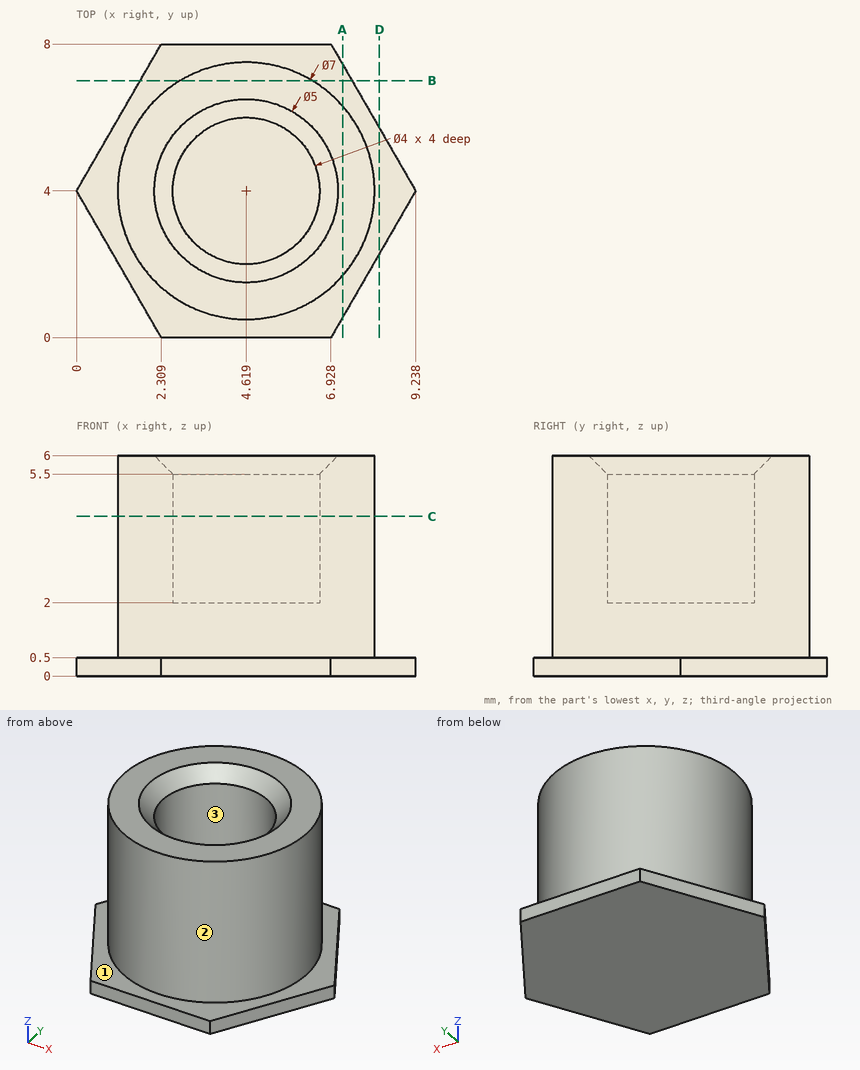
The figure shows three views and two pictorial views of one solid part (mm, origin at its lowest corner). Answer the questions. Coordinates: 2 decimals unless noted, no trailing zeros. Loops run counter-clockwise (first coordinate to the right, second up) from the corner with the lowest first, then second, coordinate; pieces in that order, holes last.
1) Find section D-D on x = 8.25. Write down the section's boundary in (y, z).
2) Find the intervals of material crossed by L1, parallel to Y at x = 4.5, z = 3.9; L2, parallel to Z at x = 3.75, y = 4.5; L3, parallel to Y at x = 5.5, z = 5.1 (1 decimal), in increasing order.
3) Find section B-B on y = 7. Write down the section's boundary in (x, z) (1 decimal), then the cut area to 3 significant figures.
4) Flat-ended cylindrical pins translate along their axes: pin 1 Ø1 at (x, y) = (4, 6) entering from +Z; pin 2 Ø1.2 at (x, y) = (5, 4) entering from +Z; pin 3 Ø1.5 at (x, z) = (1.5, 2.5) entering from +Y. Find the tip coordinate at first contact, or state that the pin passes through.
5) Find section A-A on x = 7.25. Write down the section's boundary in (y, z).
6) Determine the mould class of the marked faces 1, 2 and 3 for opening direction Y: pulls with the +Y half, pulls with the -Y half, needs draft (parallel to the pull), parting line crosses it, or undercut.
7) Find section C-C on z = 4.35. Write down the section's boundary in (x, y).
Values:
1. outline: (2.29, 0) - (5.71, 0) - (5.71, 0.5) - (2.29, 0.5) - close
2. L1: y = 0.5 to 2, 6 to 7.5
2. L2: z = 0 to 2
2. L3: y = 0.6 to 2.2, 5.8 to 7.4
3. outline: (1.7, 0) - (7.5, 0) - (7.5, 0.5) - (6.4, 0.5) - (6.4, 6) - (2.8, 6) - (2.8, 0.5) - (1.7, 0.5) - close
3. area: 22.7 mm2
4. pin 1: stops at z = 6
4. pin 2: stops at z = 2
4. pin 3: stops at y = 6.58
5. outline: (0.56, 0) - (7.44, 0) - (7.44, 0.5) - (6.31, 0.5) - (6.31, 6) - (1.69, 6) - (1.69, 0.5) - (0.56, 0.5) - close
6. face 1: needs draft
6. face 2: parting line crosses it
6. face 3: undercut
7. outline: circle Ø7 at (4.62, 4); hole circle Ø4 at (4.62, 4)
